Source: CAD feature listing. Evaluate the final solid. Frame: model axes, mm. Give positions to 0.01 mm unless a question says otherwise; leave off trailing zeros. Order: outer loops, then holes, each group sorted by start corner. A loop starts at its lowest first (then second) coordinate and runs counter-clockwise, first axis right, second up.
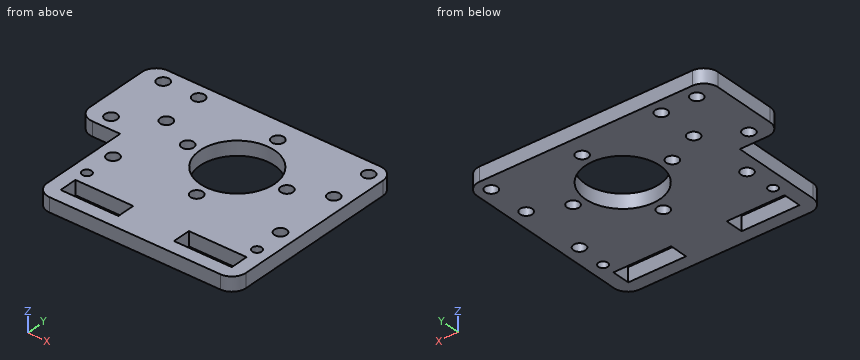
from build123d import *

# Parameters (mm, degrees)
SKETCH_1_W          = 70
SKETCH_1_H          = 69
SKETCH_1_R          = 1.65
SKETCH_1_W_2        = 20.4
SKETCH_1_H_2        = 6.4
SKETCH_1_R_2        = 2.15
SKETCH_1_R_3        = 13.15
SKETCH_1_W_3        = 15
EXTRUDE_1_DEPTH     = 5
SKETCH_2_W          = 14.8
SKETCH_2_H          = 36.5
CUT_EXTRUDE_1_DEPTH = 67.790717918
FILLET_1_R          = 5


with BuildPart() as part:
    # ｽｹｯﾁ1 → ﾎﾞｽ - 押し出し1 (new body)
    # profile 1 of 2: a face of its own
    with BuildSketch(Plane.XY):
        with Locations((0, -9.5)):
            Rectangle(SKETCH_1_W, SKETCH_1_H)
        with Locations((-30, -28.2)):
            Circle(SKETCH_1_R, mode=Mode.SUBTRACT)
        with Locations((-20, -36.1)):
            Rectangle(SKETCH_1_W_2, SKETCH_1_H_2, mode=Mode.SUBTRACT)
        with Locations((-29.55, -17.5)):
            Circle(SKETCH_1_R_2, mode=Mode.SUBTRACT)
        with Locations((20, -36.1)):
            Rectangle(SKETCH_1_W_2, SKETCH_1_H_2, mode=Mode.SUBTRACT)
        with Locations((30, -28.2)):
            Circle(SKETCH_1_R, mode=Mode.SUBTRACT)
        with Locations((0, -17.5)):
            Circle(SKETCH_1_R_2, mode=Mode.SUBTRACT)
        with Locations((29.55, -17.5)):
            Circle(SKETCH_1_R_2, mode=Mode.SUBTRACT)
        with Locations((-29.55, 5.5)):
            Circle(SKETCH_1_R_2, mode=Mode.SUBTRACT)
        with Locations((-17.5, 0)):
            Circle(SKETCH_1_R_2, mode=Mode.SUBTRACT)
        with Locations((-30, 20)):
            Circle(SKETCH_1_R_2, mode=Mode.SUBTRACT)
        Circle(SKETCH_1_R_3, mode=Mode.SUBTRACT)
        with Locations((17.5, 0)):
            Circle(SKETCH_1_R_2, mode=Mode.SUBTRACT)
        with Locations((29.55, 5.5)):
            Circle(SKETCH_1_R_2, mode=Mode.SUBTRACT)
        with Locations((0, 17.5)):
            Circle(SKETCH_1_R_2, mode=Mode.SUBTRACT)
        with Locations((30, 20)):
            Circle(SKETCH_1_R_2, mode=Mode.SUBTRACT)
    # profile 2 of 2: a face of its own
    with BuildSketch(Plane.XY):
        with Locations((-42.5, -9.5)):
            Rectangle(SKETCH_1_W_3, SKETCH_1_H)
        with Locations((-42.5, -2.5)):
            Circle(SKETCH_1_R_2, mode=Mode.SUBTRACT)
        with Locations((-42.5, 20)):
            Circle(SKETCH_1_R_2, mode=Mode.SUBTRACT)
    extrude(amount=EXTRUDE_1_DEPTH)

    # ｽｹｯﾁ2 → ｶｯﾄ - 押し出し1 (cut, through all)
    with BuildSketch(Plane.XY.offset(5)):
        with Locations((-42.6, -25.75)):
            Rectangle(SKETCH_2_W, SKETCH_2_H)
    extrude(amount=-CUT_EXTRUDE_1_DEPTH, mode=Mode.SUBTRACT)

    # ﾌｨﾚｯﾄ1
    fillet_1_edges = [part.edges().sort_by_distance(p)[0] for p in [
        (-50, 25, 2.5),
        (35, 25, 2.5),
        (35, -44, 2.5),
        (-50, -7.5, 2.5),
        (-35.2, -44, 2.5),
    ]]
    fillet(fillet_1_edges, radius=FILLET_1_R)


solid = part.part
1) Ray query, L1, parallel to Y at x = 0, z = 1.95; L2, parallel to Y at x = 23, z = 2.3; L3, parallel to Y at x = 29.55, z = 1.3. Return the intervals inside material, ascending.
Checks:
L1: y = -44 to -19.65, -15.35 to -13.15, 13.15 to 15.35, 19.65 to 25
L2: y = -44 to -39.3, -32.9 to 25
L3: y = -44 to -39.3, -32.9 to -29.79, -26.61 to -19.65, -15.35 to 3.35, 7.65 to 17.9, 22.1 to 25
2) Section query D-D on y = -28.2. Output: boundary loops of the cut face in (x, z).
Checks:
outline: (-35.2, 0) - (-31.65, 0) - (-31.65, 5) - (-35.2, 5) - close; (-28.35, 0) - (28.35, 0) - (28.35, 5) - (-28.35, 5) - close; (31.65, 0) - (35, 0) - (35, 5) - (31.65, 5) - close
3) Section query B-B on x = -42.5. Output: boundary loops of the cut face in (y, z), and give its area (4 significant figures).
Checks:
outline: (-7.5, 0) - (-4.65, 0) - (-4.65, 5) - (-7.5, 5) - close; (-0.35, 0) - (17.85, 0) - (17.85, 5) - (-0.35, 5) - close; (22.15, 0) - (25, 0) - (25, 5) - (22.15, 5) - close
area: 119.5 mm2
4) Section query C-C on y = -9.5. Output: boundary loops of the cut face in (x, z).
Checks:
outline: (-35.2, 0) - (-9.09, 0) - (-9.09, 5) - (-35.2, 5) - close; (9.09, 0) - (35, 0) - (35, 5) - (9.09, 5) - close
5) Section query A-A on z = 1. State how many separate pieces and enclosed holes the cut face has, and give its area (3 significant figures).
Checks:
separate pieces: 1
enclosed holes: 17
area: 4,300 mm2
6) First-contact query: pin 1 Ø2.5 at (x, y) = (17.5, 0) entering from +Z; pin 2 Ø2.5 at (y, z) = (-36.5, 1.5) entering from -X. Flat tips, straight axial feed; report the tip coordinate or a pass-through.
Checks:
pin 1: passes through
pin 2: stops at x = -35.2
